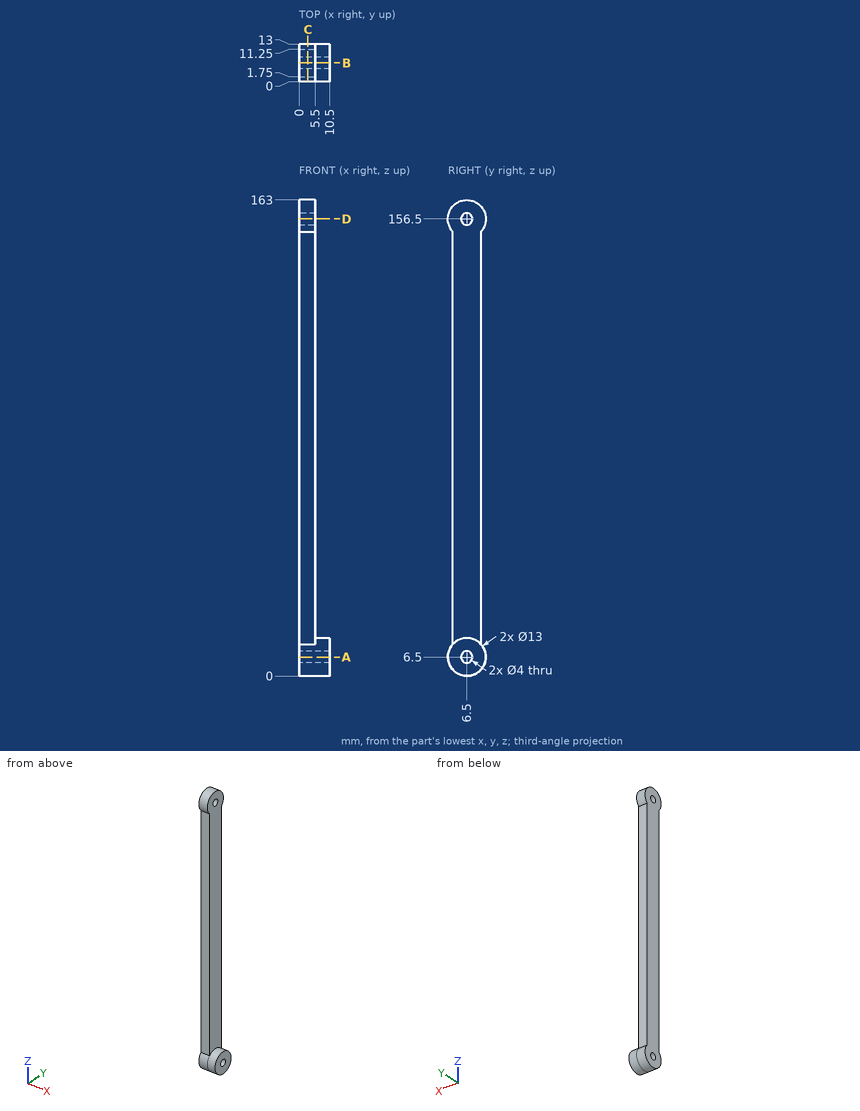
Geometry: see drawing. Coordinates: mm, zero at the bounding-box minimum. Give positions to 0.01 mm unless a question says otherwise; leave off trailing zeros. Order: outer loops, then holes, each group sorted by start corner. A loop starts at its lowest first (then second) coordinate and runs counter-clockwise, first axis right, second up.
Q1. Ray query, probe 1 along Y at (x, z) = (7.5, 6.5); probe 2 along X at (y, z) = (4.75, 104); probe 3 along Y at (x, z) = (4, 91). Return the intervals inside material, ascending.
Checked values:
probe 1: y = 0 to 4.5, 8.5 to 13
probe 2: x = 0 to 5.5
probe 3: y = 1.75 to 11.25
Q2. Section C-C on x = 3. Output: boundary loops of the cut face in (y, z).
Checked values:
outline: (1.75, 10.94) arc R6.5 ccw (long way) to (11.25, 10.94) - (11.25, 152.06) arc R6.5 ccw (long way) to (1.75, 152.06) - close; hole circle Ø4 at (6.5, 6.5); hole circle Ø4 at (6.5, 156.5)
Q3. Contact query for flat-ended pins moving along their axis: pin 1 Ø1.6 at (x, z) = (2.5, 79) entering from +Y; pin 2 Ø6.5 at (y, z) = (6.5, 156.5) entering from +X; pin 3 Ø1 at (x, y) = (4.5, 11.5) entering from +Z. Output: stop coordinate, or through.
Checked values:
pin 1: stops at y = 11.25
pin 2: stops at x = 5.5
pin 3: stops at z = 161.19
Q4. Section B-B on y = 6.5. Output: boundary loops of the cut face in (x, z), and give its area (4 significant figures).
Checked values:
outline: (0, 0) - (10.5, 0) - (10.5, 4.5) - (0, 4.5) - close; (0, 8.5) - (10.5, 8.5) - (10.5, 13) - (5.5, 13) - (5.5, 154.5) - (0, 154.5) - close; (0, 158.5) - (5.5, 158.5) - (5.5, 163) - (0, 163) - close
area: 897.5 mm2
Q5. Section A-A on z = 6.5. Output: boundary loops of the cut face in (x, y), and give its area (3 significant figures).
Checked values:
outline: (0, 0) - (10.5, 0) - (10.5, 4.5) - (0, 4.5) - close; (0, 8.5) - (10.5, 8.5) - (10.5, 13) - (0, 13) - close
area: 94.5 mm2
Q6. Section D-D on z = 156.5. Output: boundary loops of the cut face in (x, y), and give its area (3 significant figures).
Checked values:
outline: (0, 0) - (5.5, 0) - (5.5, 4.5) - (0, 4.5) - close; (0, 8.5) - (5.5, 8.5) - (5.5, 13) - (0, 13) - close
area: 49.5 mm2
